Part model, mm, in its own coordinate system. Face numbers are marked on the shaded views. A direction names the side the tool comes from. Round coordinates to 2 decimals unless told otherwise and drop trailing zeros. Order: outer loops, then holes, each group sorted by start corner. A loop starts at its lowest first (then second) coordinate and runs counter-clockwise, first axis right, second up. Notation, with made-up numbers: (89.5, -4.75) -> (98.5, -4.75) arc R20 ccw to (98.5, 21.25) -> close; hole circle Ø1 at (86, 40.5). An arc over 180 degrees is marked (long way). Return JSON: item names as keys, results as strings. Group by question number.
from build123d import *

# Parameters (mm, degrees)
BOSS_EXTRUDE1_START = 25
BOSS_EXTRUDE1_DEPTH = 50
SKETCH2_R           = 1.75
CUT_EXTRUDE1_DEPTH  = 35.321312345
CUT_EXTRUDE2_START  = -5
CUT_EXTRUDE2_DEPTH  = 10
CHAMFER1_SIZE       = 2
CHAMFER2_SIZE       = 1
FILLET1_R           = 2
FILLET3_R           = 2
CHAMFER4_SIZE       = 0.4
FILLET2_R           = 2
CHAMFER5_SIZE       = 0.4


with BuildPart() as part:
    # Sketch1 → Boss-Extrude1 (new body)
    with BuildSketch(Plane(origin=(0, 0, 0), x_dir=(1, 0, 0), z_dir=(0, 1, 0)).offset(BOSS_EXTRUDE1_START)):
        with BuildLine():
            Line((-21.040496218, 41), (-10.535653753, 41))
            ThreePointArc((-10.535653753, 41), (0, 38), (10.535653753, 41))
            Line((10.535653753, 41), (21.040496218, 41))
            Line((21.040496218, 41), (21.040496218, 33))
            Line((21.040496218, 33), (6.614378278, 33))
            ThreePointArc((6.614378278, 33), (0, 30.5), (-6.614378278, 33))
            Line((-6.614378278, 33), (-21.040496218, 33))
            Line((-21.040496218, 33), (-21.040496218, 41))
        make_face()
    extrude(amount=-BOSS_EXTRUDE1_DEPTH)

    # Sketch2 → Cut-Extrude1 (cut, through all)
    with BuildSketch(Plane(origin=(0, 0, -41), x_dir=(-1, 0, 0), z_dir=(0, 0, -1))):
        with Locations((-16, 20)):
            Circle(SKETCH2_R)
        with Locations((16, 20)):
            Circle(SKETCH2_R)
        with Locations((-16, -20)):
            Circle(SKETCH2_R)
        with Locations((16, -20)):
            Circle(SKETCH2_R)
    extrude(amount=-CUT_EXTRUDE1_DEPTH, mode=Mode.SUBTRACT)

    # Sketch3 → Cut-Extrude2 (cut)
    with BuildSketch(Plane(origin=(0, 0, 0), x_dir=(1, 0, 0), z_dir=(0, 1, 0)).offset(CUT_EXTRUDE2_START)):
        with BuildLine():
            Line((-21.040496218, 41), (-21.040496218, 8.382266622))
            Line((-21.040496218, 8.382266622), (21.040496218, 8.382266622))
            Line((21.040496218, 8.382266622), (21.040496218, 41))
            Line((21.040496218, 41), (12.961481397, 41))
            Line((12.961481397, 41), (12.961481397, 39))
            ThreePointArc((12.961481397, 39), (0, 35), (-12.961481397, 39))
            Line((-12.961481397, 39), (-12.961481397, 41))
            Line((-12.961481397, 41), (-21.040496218, 41))
        make_face()
    cut_extrude2 = extrude(amount=-CUT_EXTRUDE2_DEPTH, mode=Mode.SUBTRACT)

    # Mirror1: Cut-Extrude2 across plane
    add(cut_extrude2.mirror(Plane.ZX), mode=Mode.SUBTRACT)

    # Chamfer1
    chamfer1_edges = [part.edges().sort_by_distance(p)[0] for p in [
        (-14.25, 20, -41),
        (17.75, -20, -41),
        (-14.25, -20, -41),
        (17.75, 20, -41),
    ]]
    chamfer(chamfer1_edges, length=CHAMFER1_SIZE)

    # Chamfer2
    chamfer2_edges = [part.edges().sort_by_distance(p)[0] for p in [
        (0, -25, -38),
        (0, 25, -38),
    ]]
    chamfer(chamfer2_edges, length=CHAMFER2_SIZE)

    # Fillet1
    fillet1_edges = [part.edges().sort_by_distance(p)[0] for p in [
        (-21.040496218, 25, -37),
        (21.040496218, 25, -37),
        (-21.040496218, -25, -37),
        (21.040496218, -25, -37),
        (-21.040496218, -15, -37),
        (21.040496218, -15, -37),
        (21.040496218, -5, -37),
        (-21.040496218, -5, -37),
        (21.040496218, 5, -37),
        (21.040496218, 15, -37),
        (-21.040496218, 5, -37),
        (-21.040496218, 15, -37),
    ]]
    fillet(fillet1_edges, radius=FILLET1_R)

    # Fillet3
    fillet3_edges = [part.edges().sort_by_distance(p)[0] for p in [
        (-12.961481397, -10, -39),
        (12.961481397, -10, -39),
        (12.961481397, 10, -39),
        (-12.961481397, 10, -39),
    ]]
    fillet(fillet3_edges, radius=FILLET3_R)

    # Chamfer4
    chamfer4_edges = [part.edges().sort_by_distance(p)[0] for p in [
        (-21.040496218, 20, -33),
        (-12.827437248, 15, -33),
        (-12.827437248, 25, -33),
        (-20.45470978, 24.414213562, -33),
        (-20.45470978, 15.585786438, -33),
        (-12.827437248, 5, -33),
        (-21.040496218, 0, -33),
        (-20.45470978, -4.414213562, -33),
        (-20.45470978, 4.414213562, -33),
        (12.827437248, -5, -33),
        (12.827437248, -15, -33),
        (-21.040496218, -20, -33),
        (-12.827437248, -25, -33),
        (-20.45470978, -24.414213562, -33),
        (-20.45470978, -15.585786438, -33),
        (21.040496218, -20, -33),
        (20.45470978, -15.585786438, -33),
        (20.45470978, -24.414213562, -33),
        (21.040496218, 0, -33),
        (20.45470978, 4.414213562, -33),
        (20.45470978, -4.414213562, -33),
        (21.040496218, 20, -33),
        (20.45470978, 24.414213562, -33),
        (20.45470978, 15.585786438, -33),
        (12.827437248, 25, -33),
        (0, 25, -30.5),
        (12.827437248, -25, -33),
        (0, -25, -30.5),
        (0, -15, -30.5),
        (-12.827437248, -5, -33),
        (-12.827437248, -15, -33),
        (0, -5, -30.5),
        (0, 15, -30.5),
        (12.827437248, 5, -33),
        (12.827437248, 15, -33),
        (0, 5, -30.5),
    ]]
    chamfer(chamfer4_edges, length=CHAMFER4_SIZE)

    # Fillet2
    fillet2_edges = [part.edges().sort_by_distance(p)[0] for p in [
        (0, 5, -35),
        (0, 15, -35),
        (0, -5, -35),
        (0, -15, -35),
        (-12.961481397, -5, -40.543913723),
        (-12.961481397, -15, -40.543913723),
        (-12.961481397, 5, -40.543913723),
        (-12.961481397, 15, -40.543913723),
        (12.706173521, 5, -39.110049665),
        (12.706173521, 15, -39.110049665),
        (12.706173521, -5, -39.110049665),
        (12.706173521, -15, -39.110049665),
        (-12.706173521, -5, -39.110049665),
        (-12.706173521, -15, -39.110049665),
        (-12.706173521, 5, -39.110049665),
        (-12.706173521, 15, -39.110049665),
        (12.961481397, -15, -40.543913723),
        (12.961481397, -5, -40.543913723),
        (12.961481397, 5, -40.543913723),
        (12.961481397, 15, -40.543913723),
    ]]
    fillet(fillet2_edges, radius=FILLET2_R)

    # Chamfer5
    chamfer5_edges = [part.edges().sort_by_distance(p)[0] for p in [
        (-15.684662112, -25, -41),
        (-20.45470978, -24.414213562, -41),
        (-21.040496218, -20, -41),
        (-20.45470978, -15.585786438, -41),
        (-17.000988807, -15, -41),
        (-13.547267834, -14.414213562, -41),
        (-12.961481397, -10, -41),
        (-13.547267834, -5.585786438, -41),
        (-17.000988807, -5, -41),
        (-20.45470978, -4.414213562, -41),
        (-21.040496218, 0, -41),
        (-20.45470978, 4.414213562, -41),
        (-17.000988807, 5, -41),
        (-13.547267834, 5.585786438, -41),
        (-12.961481397, 10, -41),
        (-13.547267834, 14.414213562, -41),
        (-17.000988807, 15, -41),
        (-20.45470978, 15.585786438, -41),
        (-21.040496218, 20, -41),
        (-20.45470978, 24.414213562, -41),
        (-15.684662112, 25, -41),
        (15.684662112, -25, -41),
        (20.45470978, -24.414213562, -41),
        (21.040496218, -20, -41),
        (20.45470978, -15.585786438, -41),
        (17.000988807, -15, -41),
        (13.547267834, -14.414213562, -41),
        (12.961481397, -10, -41),
        (13.547267834, -5.585786438, -41),
        (17.000988807, -5, -41),
        (20.45470978, -4.414213562, -41),
        (21.040496218, 0, -41),
        (20.45470978, 4.414213562, -41),
        (17.000988807, 5, -41),
        (13.547267834, 5.585786438, -41),
        (12.961481397, 10, -41),
        (13.547267834, 14.414213562, -41),
        (17.000988807, 15, -41),
        (20.45470978, 15.585786438, -41),
        (21.040496218, 20, -41),
        (20.45470978, 24.414213562, -41),
        (15.684662112, 25, -41),
    ]]
    chamfer(chamfer5_edges, length=CHAMFER5_SIZE)


solid = part.part
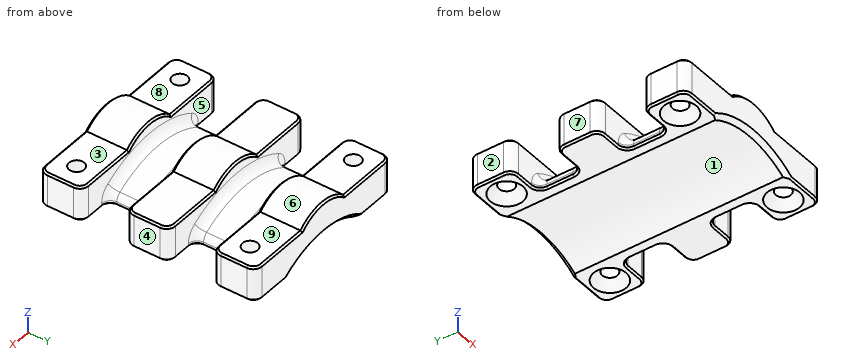
(1) Probe L1, parallel to Y at x = 16, z = -36.2; L2, parallel to Y at x = -8, z = -33.5; L3, parallel to Y at x = 0, z = -33.75. List the from-to ranges inside material, lowest first. Write a range as [from, to].
(2) Tool access for the marked faces 5, 6, 7, 8 and 9: list every direction of +Z, -Z, +X, -X, +Y, -Y with a clear straight run to the whole face (end or side of a thin tool).
(3) Pin check, flat tips, straight feed: P1, Ø10, axis at x = -12.5, y = 19, coming from the +Z side; P2, Ø0.6, axis at y = 9.5, z = -40.5, coming from the -X side. Stop position of each tip, or through.
(4) Saw through at B-B, the plane x = 16. State how many separate pieces and enclosed holes the cut face has, and give its area (3 significant figures).
(5) Saw through at A-A, the plane y = 20. List the corners of the cut face in (x, z).
(6) Saw through at C-C, the plane y = -9. List the corners of the cut face in (x, z), and give its area (3 significant figures).
(7) Mould opens along X. For the marked faces 1, 2, 3 and 4 say: pulls with the +X half, pulls with the -X half, needs draft (parallel to the pull), parting line crosses it, or undercut.
Results are:
{
 "1": {"L1": "y = [-25, -21.75], [-18.25, -15], [-5, 5], [15, 18.25], [21.75, 25]", "L2": "y = [-25, -15], [-5, 5], [15, 25]", "L3": "y = [-25, -14.85], [-5.15, 5.15], [14.85, 25]"},
 "2": {"face 5": "+Z", "face 6": "+Z, +Y, -Y", "face 7": "+Z, -Z, -X, +Y, -Y", "face 8": "+Z, -X, +Y, -Y", "face 9": "+Z, +X, +Y, -Y"},
 "3": {"P1": "stops at z = -33", "P2": "stops at x = -12.96"},
 "4": {"separate pieces": "5", "enclosed holes": "0", "area": "175 mm^2"},
 "5": {"outline": "(-21.04, -40.6) -> (-20.64, -41) -> (-19.75, -41) -> (-17.75, -39) -> (-17.75, -33) -> (-20.64, -33) -> (-21.04, -33.4) -> close; (-14.25, -39) -> (-12.25, -41) -> (-10.54, -41) arc R20 cw to (10.54, -41) -> (12.25, -41) -> (14.25, -39) -> (14.25, -33) -> (6.61, -33) arc R10 ccw to (-6.61, -33) -> (-14.25, -33) -> close; (17.75, -39) -> (19.75, -41) -> (20.64, -41) -> (21.04, -40.6) -> (21.04, -33.4) -> (20.64, -33) -> (17.75, -33) -> close"},
 "6": {"outline": "(-12.96, -40.6) -> (-12.56, -41) -> (-10.54, -41) arc R20 cw to (10.54, -41) -> (12.56, -41) -> (12.96, -40.6) -> (12.96, -40.09) arc R2 ccw to (12.01, -38.38) arc R23 ccw to (-12.01, -38.38) arc R2 ccw to (-12.96, -40.09) -> close", "area": "78.9 mm^2"},
 "7": {"face 1": "undercut", "face 2": "pulls with the -X half", "face 3": "needs draft", "face 4": "pulls with the +X half"}
}
